Design review of the part built by this model. Coordinates are the model's own, in mm. A direction names the side the tool comes from. Coordinates: 2 decimals unless noted, no trailing zeros. Loops run counter-clockwise (first coordinate to the right, second up) from the corner with the lowest first, then second, coordinate; pieces in that order, holes last. Notation, with made-up numbers: (57.25, 19.5) - (115.25, 19.5) arc R12 cw to (115.25, 30.5) - close; hole circle Ø8 at (-26, 10.25). An arc over 180 degrees is marked (long way). Answer in a Markdown table with one row per item. Add a question column.
(1) We need section C-C, the plane z = 11.5. Write out the cut boundary in (x, y).
(2) Clearance check with flat-ended pins moving along their axes: pin 1 (12 mm diameter, centred on x = 39.5, z = 21, fed in from +Y); pin 2 (6 mm diameter, centred on x = -11.47, y = -60.93, fed in from -Z); pin 3 (23.5 mm diameter, centred on x = 11.47, y = 60.93, fed in from +Z); pin 4 (10.5 mm diameter, centred on x = 58.5, y = 20.53, fed in from +Z). State where each tip first meets the part, or that it passes through.
(3) We need section A-A, the plane y = 0. Write out the cut boundary in (x, z), plus the area to 3 significant figures.
(4) For faces 1 (the face through (64.274, 16.105, 0.493)), 2 (the face through (-69.15, -21.78, 3.55)), 3 (the face through (38, -38, 7)), list the 3-axis set-ups (+Z, -Z, +X, -X, +Y, -Y) from which the entire face can be reached by the end or side of a thin tool; tool diameter is ignored.
(5) We need section D-D, the plane z = 52. Write out the cut boundary in (x, y).
(6) The part is to be moulded in two halves that separate along X. For faces 4 (the face through (11, -19, 57)), 5 (the face through (-50.076, -15.77, 17.14)), 6 (the face through (-43.983, 39.135, 4.042)), say which applies: released by +X, released by -X, zero draft, split by the parting line, or undercut.
(7) To check wall thickness, follow L1, parallel to X at y = -17.5, z = 3; L2, parallel to Z at x = -33, y = 23; L3, parallel to Z at x = -21.5, y = -62.5. State the ranges of each line that lie inside material, in increasing order. Write a range as [from, to].
from build123d import *

# Parameters (mm, degrees)
FILLET1_R                               = 12
CBORE_FOR_M6_HEX_HEAD_BOLT1_D           = 6.6
CBORE_FOR_M6_HEX_HEAD_BOLT1_CBORE_D     = 14.547
CBORE_FOR_M6_HEX_HEAD_BOLT1_CBORE_DEPTH = 1
CIRPATTERN1_COUNT                       = 6


with BuildPart() as part:
    # Sketch2 → Revolve1 (revolve)
    with BuildSketch(Plane(origin=(0, 0, 0), x_dir=(1, 0, 0), z_dir=(0, 1, 0))):
        Polygon((-72.5, 0), (-72.5, -7), (-52.5, -7), (-52.5, -27), (-25, -27), (-25, -57), (-21.63, -57), (-21.63, 0), align=None)
    revolve(axis=Axis((0, 0, 0), (0, 0, 1)))

    # Fillet1
    fillet1_edges = [part.edges().sort_by_distance(p)[0] for p in [
        (25, 0, 27),
    ]]
    fillet(fillet1_edges, radius=FILLET1_R)

    # CBORE for M6 Hex Head Bolt1 (through all)
    with Locations(Plane(origin=(-47.031359199, 40.398654085, 0), x_dir=(-1, 0, 0), z_dir=(0, 0, -1))):
        with Locations((0, 0)):
            cbore_for_m6_hex_head_bolt1 = CounterBoreHole(CBORE_FOR_M6_HEX_HEAD_BOLT1_D / 2, CBORE_FOR_M6_HEX_HEAD_BOLT1_CBORE_D / 2, CBORE_FOR_M6_HEX_HEAD_BOLT1_CBORE_DEPTH)

    # CirPattern1: CBORE for M6 Hex Head Bolt1 ×6 about axis
    cirpattern1_axis = Axis((0, 0, 0), (0, 0, 1))
    for i in range(1, CIRPATTERN1_COUNT):
        add(cbore_for_m6_hex_head_bolt1.rotate(cirpattern1_axis, i * 360 / CIRPATTERN1_COUNT), mode=Mode.SUBTRACT)


solid = part.part
Responses:
| question | item | result |
|---|---|---|
| 1 | outline | circle Ø105 at (0, 0); hole circle Ø43.26 at (0, 0) |
| 2 | pin 1 | stops at y = 40.42 |
| 2 | pin 2 | passes through |
| 2 | pin 3 | stops at z = 27 |
| 2 | pin 4 | stops at z = 7 |
| 3 | outline | (-72.5, 0) - (-21.63, 0) - (-21.63, 57) - (-25, 57) - (-25, 39) arc R12 cw to (-37, 27) - (-52.5, 27) - (-52.5, 7) - (-72.5, 7) - close; (21.63, 0) - (72.5, 0) - (72.5, 7) - (52.5, 7) - (52.5, 27) - (37, 27) arc R12 cw to (25, 39) - (25, 57) - (21.63, 57) - close |
| 3 | area | 2,210 mm2 |
| 4 | face 1 | -Z |
| 4 | face 2 | +Z, -Z |
| 4 | face 3 | +Z |
| 5 | outline | circle Ø50 at (0, 0); hole circle Ø43.26 at (0, 0) |
| 6 | face 4 | zero draft |
| 6 | face 5 | split by the parting line |
| 6 | face 6 | undercut |
| 7 | L1 | x = [-70.36, -59.81], [-57.2, -12.71], [12.71, 70.36] |
| 7 | L2 | z = [0, 27] |
| 7 | L3 | z = [0, 7] |
